CAD build for the part. Positions are in the model's coordinates, mm. A direction names the side the tool comes from. Round coordinates to 2 decimals unless told otherwise and drop trailing zeros. Order: outer loops, then holes, each group sorted by start corner. A loop starts at its lowest first (then second) coordinate and runs counter-clockwise, first axis right, second up.
```python
from build123d import *

# Parameters (mm, degrees)
F0_W     = 50
F0_H     = 5
F1_DEPTH = 5
F2_W     = 2.8276949842
F2_H     = 15
F3_DEPTH = 5.1


with BuildPart() as f1:
    # F0 (on Right) → F1 (new body)
    with BuildSketch(Plane.YZ):
        with Locations((-7.4186130613, -1.9997399262)):
            Rectangle(F0_W, F0_H)
    extrude(amount=F1_DEPTH)

    # F2 (on face) → F3 (cut)
    with BuildSketch(Plane(origin=(0, 0, -4.4997399262), x_dir=(1, 0, 0), z_dir=(0, 0, -1))):
        with Locations((3.5861525079, 19.9186130613)):
            Rectangle(F2_W, F2_H)
        with Locations((3.5861525079, -5.0813869387)):
            Rectangle(F2_W, F2_H)
    extrude(amount=-F3_DEPTH, mode=Mode.SUBTRACT)


solid = f1.part
```
1. Pin check, flat tip, straight feed: P1, Ø2, axis at y = 11, z = -3.5, coming from the +X side. Stop position of the tip, or through.
2. Mould opens along Y. For faces 3 (the face through (2, -8, 0.5)), 4 (the face through (4, -12.419, -2)), 5 (the face through (2, -32.419, -2)) say: released by +Y, released by -Y, zero draft, split by the parting line, or undercut.
3. Cut at B-B, the plane z = 0.05. Write the cut outline in (x, y).
4. Drill centre lines: line 1 (Y direction, x = 3.9, z = -0.85); line 2 (X direction, y = -1.5, z = -3.8). Where is each one in solid material? Low to high.
5. Cut at C-C, the plane y = -13. Write the cut outline in (x, z).
6. Cut at A-A, the plane x = 3.05. Write the cut outline in (y, z), and give its area (3 significant figures).
7. Tool access for faces 1 (the face through (2, -8, -4.5)), 2 (the face through (4, 12.581, -2)): list every direction of +Z, -Z, +X, -X, +Y, -Y with a clear straight run to the whole face (end or side of a thin tool).
Outcome:
1. P1: stops at x = 2.17
2. face 3: zero draft
2. face 4: undercut
2. face 5: released by -Y
3. outline: (0, -32.42) - (5, -32.42) - (5, -27.42) - (2.17, -27.42) - (2.17, -12.42) - (5, -12.42) - (5, -2.42) - (2.17, -2.42) - (2.17, 12.58) - (5, 12.58) - (5, 17.58) - (0, 17.58) - close
4. line 1: y = -32.42 to -27.42, -12.42 to -2.42, 12.58 to 17.58
4. line 2: x = 0 to 2.17
5. outline: (0, -4.5) - (2.17, -4.5) - (2.17, 0.5) - (0, 0.5) - close
6. outline: (-32.42, -4.5) - (-27.42, -4.5) - (-27.42, 0.5) - (-32.42, 0.5) - close; (-12.42, -4.5) - (-2.42, -4.5) - (-2.42, 0.5) - (-12.42, 0.5) - close; (12.58, -4.5) - (17.58, -4.5) - (17.58, 0.5) - (12.58, 0.5) - close
6. area: 100 mm2
7. face 1: -Z, +X, -X, +Y, -Y
7. face 2: +Z, -Z, +X
